Geometry check sheet. Reference: drawing and pictorial views, mm from the part's lowest x, y, z. A direction names the side the tool comes from. Give positions to 0.01 mm unless a question says otherwise; leave off trailing zeros. Order: outer loops, then holes, each group sorted by start corner. A loop starts at its lowest first (then second) coordinate and runs counter-clockwise, first axis right, second up.
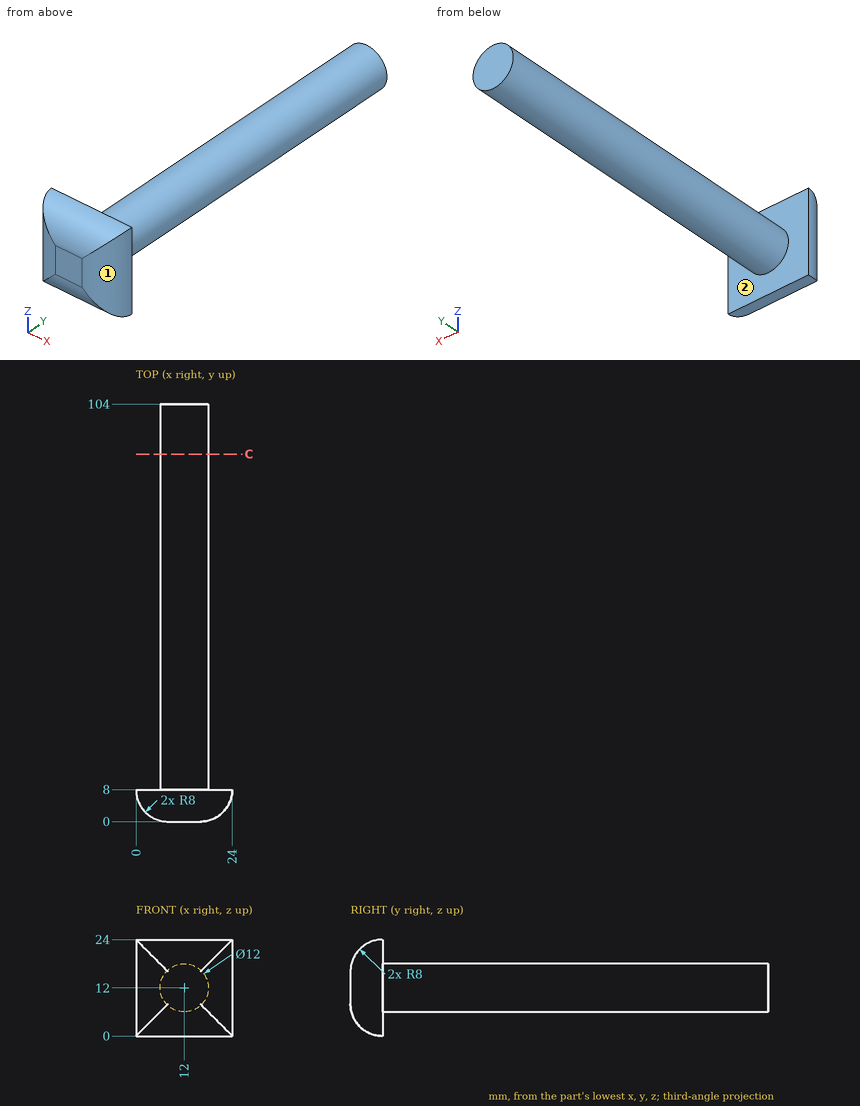
(1) Material ranges on L1, parallel to X at y = 99.5, z = 12.5; L2, parallel to X at y = 97.5, z = 16; L3, parallel to Z at x = 11.75, y = 36 (3 decimals), recorded low to high.
Response values:
L1: x = 6.02 to 17.98
L2: x = 7.53 to 16.47
L3: z = 6.005 to 17.995
(2) Gauge pin test, flat ends, axial feed: pin 1 Ø5 at (x, y) = (15, 83.5) entering from +Z; pin 2 Ø8 at (x, y) = (11.5, 84) entering from -Z; pin 3 Ø12 at (y, z) = (57.5, 6.5) entering from +X. Record the tip position at first contact, or that the pin passes through.
Response values:
pin 1: stops at z = 17.98
pin 2: stops at z = 6
pin 3: stops at x = 18
(3) Set-up check for the marked faces 1 and 2: record each of +Z, -Z, +X, -X, +Y, -Y from which the full face is reachable in a straight line by a thin tool's end or side.
Response values:
face 1: +Z, -Z, +X, -Y
face 2: +Y
(4) Cross-section at C-C on y = 91.5. Enter the section's corners in (x, z), then the cut area to 3 significant figures.
Response values:
outline: circle Ø12 at (12, 12)
area: 113 mm2
